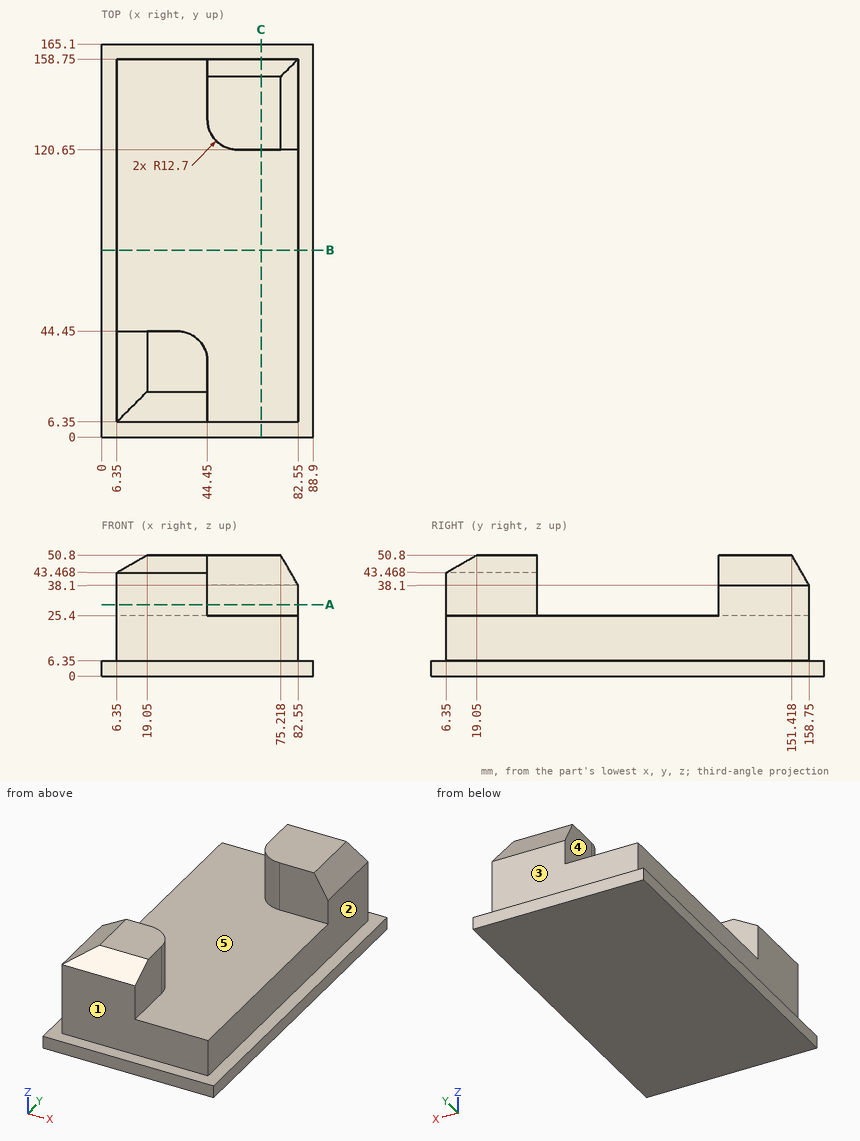
The drawing under review shows one solid part. Ordinate dimensions are in mm from its lowest x, y, z. A direction names the side the tool comes from. Round coordinates to 2 decimals unless told otherwise and drop trailing zeros. Write each loop counter-clockwise with the first axis right and the second up, starting at its lowest first coordinate (ties: lowest second). Pieces come first, ordered by that corner, then holes.
(1) Insertion check: pin 1 (12.5 mm diameter, centred on x = 66, z = 41, fed in from -Y); pin 2 (20.5 mm diameter, centred on y = 23, z = 38.5, fed in from +X); pin 3 (1 mm diameter, centred on y = 111.5, z = 7, fed in from -X). Each pin has a flat end and moves straight along its axis. Give the tip position at first contact, or say it passes through.
(2) We need section A-A on z = 30. Give the boundary of the cut face in (x, y).
(3) Machinability: for the marked faces 1, 2, 3, 4 and 5, which of the approach directions +Z, -Z, +X, -X, +Y, -Y give a long, thin tool a straight path to every point of the face, cutting with its end or side? Answer none if there is none.
(4) We need section C-C on x = 67. Give the boundary of the cut face in (y, z).
(5) Wall thickness on L1, parallel to Z at x = 79.5, y = 28; L2, parallel to Y at x = 20, z = 31; L3, parallel to X at y = 17.5, z = 11.5: over which ranges is each line inside the solid? List them lowest first.
(6) We need section B-B on y = 78.5. Give the boundary of the cut face in (x, z), and give its area (3 significant figures).
Findings below:
1. pin 1: stops at y = 120.65
1. pin 2: stops at x = 44.45
1. pin 3: stops at x = 6.35
2. outline: (6.35, 6.35) - (44.45, 6.35) - (44.45, 31.75) arc R12.7 ccw to (31.75, 44.45) - (6.35, 44.45) - close; (44.45, 133.35) arc R12.7 ccw to (57.15, 120.65) - (82.55, 120.65) - (82.55, 158.75) - (44.45, 158.75) - close
3. face 1: +Z, +X, -X, -Y
3. face 2: +Z, +X, +Y, -Y
3. face 3: +Z, +X, -X, +Y
3. face 4: +Z, -X, +Y
3. face 5: +Z
4. outline: (0, 0) - (165.1, 0) - (165.1, 6.35) - (158.75, 6.35) - (158.75, 38.1) - (151.42, 50.8) - (120.65, 50.8) - (120.65, 25.4) - (6.35, 25.4) - (6.35, 6.35) - (0, 6.35) - close
5. L1: z = 0 to 25.4
5. L2: y = 6.35 to 44.45
5. L3: x = 6.35 to 82.55
6. outline: (0, 0) - (88.9, 0) - (88.9, 6.35) - (82.55, 6.35) - (82.55, 25.4) - (6.35, 25.4) - (6.35, 6.35) - (0, 6.35) - close
6. area: 2,020 mm2
